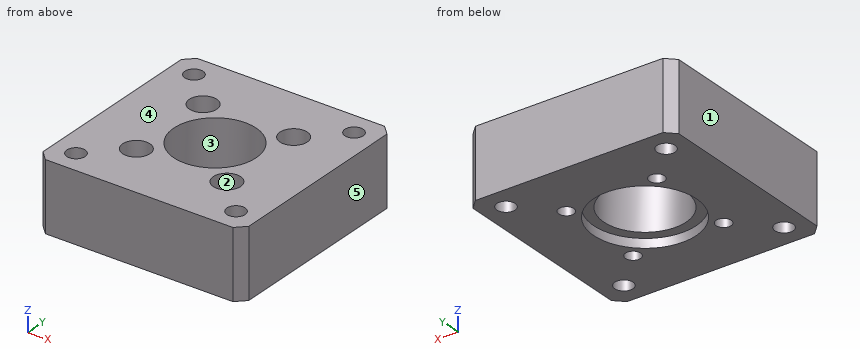
from build123d import *

# Parameters (mm, degrees)
SKETCH1_W           = 45
SKETCH1_H           = 45
SKETCH1_R           = 9
SKETCH1_R_2         = 2
BOSS_EXTRUDE1_DEPTH = 15
SKETCH2_R           = 1.65
CUT_EXTRUDE1_DEPTH  = 15
SKETCH3_R           = 3
CUT_EXTRUDE2_DEPTH  = 8
CHAMFER1_SIZE       = 2
SKETCH4_R           = 11.2
CUT_EXTRUDE3_DEPTH  = 2


with BuildPart() as part:
    # Sketch1 → Boss-Extrude1 (new body)
    with BuildSketch(Plane.XY):
        Rectangle(SKETCH1_W, SKETCH1_H)
        Circle(SKETCH1_R, mode=Mode.SUBTRACT)
        with Locations((-17.5, 17.5)):
            Circle(SKETCH1_R_2, mode=Mode.SUBTRACT)
        with Locations((17.5, 17.5)):
            Circle(SKETCH1_R_2, mode=Mode.SUBTRACT)
        with Locations((17.5, -17.5)):
            Circle(SKETCH1_R_2, mode=Mode.SUBTRACT)
        with Locations((-17.5, -17.5)):
            Circle(SKETCH1_R_2, mode=Mode.SUBTRACT)
    extrude(amount=BOSS_EXTRUDE1_DEPTH)

    # Sketch2 → Cut-Extrude1 (cut)
    with BuildSketch(Plane.XY.offset(15)):
        with Locations((9.899494937, 9.899494937)):
            Circle(SKETCH2_R)
        with Locations((9.899494937, -9.899494937)):
            Circle(SKETCH2_R)
        with Locations((-9.899494937, -9.899494937)):
            Circle(SKETCH2_R)
        with Locations((-9.899494937, 9.899494937)):
            Circle(SKETCH2_R)
    extrude(amount=-CUT_EXTRUDE1_DEPTH, mode=Mode.SUBTRACT)

    # Sketch3 → Cut-Extrude2 (cut)
    with BuildSketch(Plane.XY.offset(15)):
        with Locations((9.899494937, 9.899494937)):
            Circle(SKETCH3_R)
        with Locations((9.899494937, -9.899494937)):
            Circle(SKETCH3_R)
        with Locations((-9.899494937, -9.899494937)):
            Circle(SKETCH3_R)
        with Locations((-9.899494937, 9.899494937)):
            Circle(SKETCH3_R)
    extrude(amount=-CUT_EXTRUDE2_DEPTH, mode=Mode.SUBTRACT)

    # Chamfer1
    chamfer1_edges = [part.edges().sort_by_distance(p)[0] for p in [
        (22.5, -22.5, 7.5),
        (-22.5, -22.5, 7.5),
        (-22.5, 22.5, 7.5),
        (22.5, 22.5, 7.5),
    ]]
    chamfer(chamfer1_edges, length=CHAMFER1_SIZE)

    # Sketch4 → Cut-Extrude3 (cut)
    with BuildSketch(Plane(origin=(0, 0, 0), x_dir=(-1, 0, 0), z_dir=(0, 0, -1))):
        Circle(SKETCH4_R)
    extrude(amount=-CUT_EXTRUDE3_DEPTH, mode=Mode.SUBTRACT)


solid = part.part
Here's how the part is built. I have some questions about the finished solid (model axes, mm). Face numbers are marked on the shaded views. A direction names the side the tool comes from. Round coordinates to 2 decimals unless told otherwise and drop trailing zeros. Order: outer loops, then holes, each group sorted by start corner. A loop starts at its lowest first (then second) coordinate and runs counter-clockwise, first axis right, second up. Notation, with made-up numbers: M 40.5,40.5 L 85.5,40.5 A28 cw 85.5,71.5 Z; hole C -16,12 d10. An arc over 180 degrees is marked long. Return JSON: item names as keys, results as strings. Group by question number.
1. If we mould it in two halves opening along X, with no side actions, what happens to the marked faces 3, 4 and 5? For each: pulls with the +X half, pulls with the -X half, needs draft (parallel to the pull), parting line crosses it, or undercut.
2. Please list where these lines run through material, in increasing order: probe 1 along X at (y, z) = (-18, 6.25); probe 2 along Y at (x, z) = (-7.5, 7.75); probe 3 along X at (y, z) = (-16, 10.25).
3. If we section it at B-B on y = 17.5: List the corners of the cut face in (x, z) for me.
4. I'm going to push flat-ended pins straight in: pin 1 Ø3 at (x, y) = (9.9, -9.9) entering from -Z; pin 2 Ø3 at (x, y) = (9, -9.5) entering from +Z. Where does each tip first touch, or does it pass through?
5. On a 3-axis mill with a long thin cutter (end or side, diameter ignored), from which of +Z, -Z, +X, -X, +Y, -Y can I reach the whole of each face in a straight line? I mean the marked faces 1 and 2. Say none if no direction works.
6. If we section it at A-A on x = 0: List the corners of the cut face in (y, z) for me, then the cut area to 3 significant figures.
7. If we section it at D-D on z = 5.75: State how many separate pieces and enclosed holes the cut face has, then the cut area to 3 significant figures.
Reply:
{
 "1": {"face 3": "undercut", "face 4": "needs draft", "face 5": "pulls with the +X half"},
 "2": {"probe 1": "-22.5 to -19.44, -15.56 to 15.56, 19.44 to 22.5", "probe 2": "-22.5 to -11.7, -8.1 to -4.97, 4.97 to 8.1, 11.7 to 22.5", "probe 3": "-22.5 to -18.82, -16.18 to 16.18, 18.82 to 22.5"},
 "3": {"outline": "M -22.5,0 L -19.5,0 L -19.5,15 L -22.5,15 Z; M -15.5,0 L 15.5,0 L 15.5,15 L -15.5,15 Z; M 19.5,0 L 22.5,0 L 22.5,15 L 19.5,15 Z"},
 "4": {"pin 1": "through", "pin 2": "z = 7"},
 "5": {"face 1": "+Z, -Z, -X, +Y, -Y", "face 2": "+Z"},
 "6": {"outline": "M -22.5,0 L -11.2,0 L -11.2,2 L -9,2 L -9,15 L -22.5,15 Z; M 9,2 L 11.2,2 L 11.2,0 L 22.5,0 L 22.5,15 L 9,15 Z", "area": "396 mm^2"},
 "7": {"separate pieces": "1", "enclosed holes": "9", "area": "1,680 mm^2"}
}
